from build123d import *

# Parameters (mm, degrees)
EXTRUDE_1_DEPTH     = 50
SKETCH_2_R          = 4
SKETCH_2_R_2        = 1.7
CUT_EXTRUDE_1_DEPTH = 50
SKETCH_3_W          = 10
SKETCH_3_H          = 10
EXTRUDE_2_DEPTH     = 2
FILLET_1_R          = 6
FILLET_2_R          = 6
FILLET_3_R          = 3
FILLET_4_R          = 3
SKETCH_5_R          = 1.5
CUT_EXTRUDE_2_DEPTH = 23
FILLET_5_R          = 2
FILLET_6_R          = 2
FILLET_7_R          = 2
FILLET_8_R          = 2
SKETCH_7_W          = 44.35766487
SKETCH_7_H          = 5
CUT_EXTRUDE_4_DEPTH = 5
CUT_EXTRUDE_5_DEPTH = 31


with BuildPart() as part:
    # 草图1 → 凸台-拉伸1 (new body)
    with BuildSketch(Plane.XY):
        Polygon((-45, 4.380640832), (-35, 4.380640832), (-35, -2.619359168), (-5, -2.619359168), (-5, 4.380640832), (5, 4.380640832), (5, -0.619359168), (0, -0.619359168), (0, -7.619359168), (-40, -7.619359168), (-40, -0.619359168), (-45, -0.619359168), align=None)
    extrude(amount=EXTRUDE_1_DEPTH)

    # 草图2 → 切除-拉伸1 (cut)
    with BuildSketch(Plane(origin=(0, -2.619359168, 0), x_dir=(1, 0, 0), z_dir=(0, 1, 0))):
        with Locations(Location((-20, -25, 0), (0, 0, 270))):
            Circle(SKETCH_2_R)
        with Locations(Location((-20, -17.75, 0), (0, 0, 270))):
            Circle(SKETCH_2_R_2)
        with Locations(Location((-12.75, -25, 0), (0, 0, 270))):
            Circle(SKETCH_2_R_2)
        with Locations(Location((-20, -32.25, 0), (0, 0, 270))):
            Circle(SKETCH_2_R_2)
        with Locations(Location((-27.25, -25, 0), (0, 0, 270))):
            Circle(SKETCH_2_R_2)
    extrude(amount=-CUT_EXTRUDE_1_DEPTH, mode=Mode.SUBTRACT)

    # 草图3 → 凸台-拉伸2 (add)
    with BuildSketch(Plane(origin=(0, 4.380640832, 0), x_dir=(1, 0, 0), z_dir=(0, 1, 0))):
        with Locations((0, -45)):
            Rectangle(SKETCH_3_W, SKETCH_3_H)
        with Locations((-40, -45)):
            Rectangle(SKETCH_3_W, SKETCH_3_H)
        with Locations((-40, -5)):
            Rectangle(SKETCH_3_W, SKETCH_3_H)
        with Locations((0, -5)):
            Rectangle(SKETCH_3_W, SKETCH_3_H)
    extrude(amount=EXTRUDE_2_DEPTH)

    # 圆角1
    fillet_1_edges = [part.edges().sort_by_distance(p)[0] for p in [
        (-40, -7.619359168, 25),
    ]]
    fillet(fillet_1_edges, radius=FILLET_1_R)

    # 圆角2
    fillet_2_edges = [part.edges().sort_by_distance(p)[0] for p in [
        (0, -7.619359168, 25),
    ]]
    fillet(fillet_2_edges, radius=FILLET_2_R)

    # 圆角3
    fillet_3_edges = [part.edges().sort_by_distance(p)[0] for p in [
        (-5, -2.619359168, 25),
    ]]
    fillet(fillet_3_edges, radius=FILLET_3_R)

    # 圆角4
    fillet_4_edges = [part.edges().sort_by_distance(p)[0] for p in [
        (-35, -2.619359168, 25),
    ]]
    fillet(fillet_4_edges, radius=FILLET_4_R)

    # 草图5 → 切除-拉伸2 (cut)
    with BuildSketch(Plane.XZ.offset(0.619359168)):
        with Locations((2.5, 47.5)):
            Circle(SKETCH_5_R)
        with Locations(Location((2.5, 2.5, 0), (0, 0, 270))):
            Circle(SKETCH_5_R)
        with Locations((-42.5, 2.5)):
            Circle(SKETCH_5_R)
        with Locations(Location((-42.5, 47.5, 0), (0, 0, 270))):
            Circle(SKETCH_5_R)
    extrude(amount=-CUT_EXTRUDE_2_DEPTH, mode=Mode.SUBTRACT)

    # 圆角5
    fillet_5_edges = [part.edges().sort_by_distance(p)[0] for p in [
        (5, 2.880640832, 50),
    ]]
    fillet(fillet_5_edges, radius=FILLET_5_R)

    # 圆角6
    fillet_6_edges = [part.edges().sort_by_distance(p)[0] for p in [
        (5, 2.880640832, 0),
    ]]
    fillet(fillet_6_edges, radius=FILLET_6_R)

    # 圆角7
    fillet_7_edges = [part.edges().sort_by_distance(p)[0] for p in [
        (-45, 2.880640832, 0),
    ]]
    fillet(fillet_7_edges, radius=FILLET_7_R)

    # 圆角8
    fillet_8_edges = [part.edges().sort_by_distance(p)[0] for p in [
        (-45, 2.880640832, 50),
    ]]
    fillet(fillet_8_edges, radius=FILLET_8_R)

    # 草图7 → 切除-拉伸4 (cut)
    with BuildSketch(Plane.XZ.offset(7.619359168)):
        with Locations((-20.290282059, 42.5)):
            Rectangle(SKETCH_7_W, SKETCH_7_H)
        with Locations((-20.290282059, 7.5)):
            Rectangle(SKETCH_7_W, SKETCH_7_H)
    extrude(amount=-CUT_EXTRUDE_4_DEPTH, mode=Mode.SUBTRACT)

    # 草图8 → 切除-拉伸5 (cut)
    with BuildSketch(Plane(origin=(0, 6.380640832, 0), x_dir=(1, 0, 0), z_dir=(0, 1, 0))):
        Polygon((-5, -40), (-8, -40), (-35, -40), (-35, -45), (-5, -45), align=None)
        Polygon((-35, -10), (-8, -10), (-5, -10), (-5, -5), (-35, -5), align=None)
    extrude(amount=-CUT_EXTRUDE_5_DEPTH, mode=Mode.SUBTRACT)


solid = part.part
Could you check a few things on this model? Use its own coordinates, in mm. A direction names the side the tool comes from. Give positions to 0.01 mm unless a question says otherwise; leave off trailing zeros. Order: outer loops, then holes, each group sorted by start corner. A loop starts at its lowest first (then second) coordinate and runs counter-clockwise, first axis right, second up. Notation, with made-up numbers: (20, 34.25) -> (61, 34.25) arc R24 ccw to (61, 44.25) -> close; hole circle Ø9 at (-12.5, 54.25). An arc over 180 degrees is marked (long way). Return JSON: item names as keys, results as strings.
1. Imagine slicing it at B-B on x = -12.75. List the corners of the cut face in (y, z) for me, then the cut area to 3 significant figures.
Answer list:
{"outline": "(-7.62, 0) -> (-2.62, 0) -> (-2.62, 5) -> (-7.62, 5) -> close; (-7.62, 10) -> (-2.62, 10) -> (-2.62, 23.3) -> (-7.62, 23.3) -> close; (-7.62, 26.7) -> (-2.62, 26.7) -> (-2.62, 40) -> (-7.62, 40) -> close; (-7.62, 45) -> (-2.62, 45) -> (-2.62, 50) -> (-7.62, 50) -> close", "area": "183 mm2"}
2. For pin 1 Ø5 at (x, z) = (-2, 30) entering from +Y; pin 2 Ø1 at (y, z) = (-4.5, 27.5) entering from +X; pin 3 Ø4 at (y, z) = (-6, 41.5) entering from +X, each with a flat end and sliding along its axis, tell me the tip position at first contact or that it passes through.
Answer list:
{"pin 1": "stops at y = 4.38", "pin 2": "stops at x = -0.49", "pin 3": "stops at x = -0.84"}
3. On a 3-axis mill with a long thin cutter (end or side, diameter ignored), from which of +Z, -Z, +X, -X, +Y, -Y can I reach the whole of each face in a straight line? I mean faces 4 (the flat face through (-42, -0.619, 25)), 5 (the flat face through (-40, 4.381, 25)), 6 (the cylindrical face through (-5.86, -1.72, 25.21)). Say none if no direction works.
Answer list:
{"face 4": "+Z, -Z, -X, -Y", "face 5": "+X, -X, +Y", "face 6": "+Z, -Z, +Y"}
4. Imagine slicing it at C-C on z = 25. List the corners of the cut face in (x, y) for me, then the cut area to 3 significant figures.
Answer list:
{"outline": "(-45, -0.62) -> (-40, -0.62) -> (-40, -1.62) arc R6 ccw to (-34, -7.62) -> (-28.95, -7.62) -> (-28.95, -2.62) -> (-32, -2.62) arc R3 cw to (-35, 0.38) -> (-35, 4.38) -> (-45, 4.38) -> close; (-25.55, -7.62) -> (-24, -7.62) -> (-24, -2.62) -> (-25.55, -2.62) -> close; (-16, -7.62) -> (-14.45, -7.62) -> (-14.45, -2.62) -> (-16, -2.62) -> close; (-11.05, -7.62) -> (-6, -7.62) arc R6 ccw to (0, -1.62) -> (0, -0.62) -> (5, -0.62) -> (5, 4.38) -> (-5, 4.38) -> (-5, 0.38) arc R3 cw to (-8, -2.62) -> (-11.05, -2.62) -> close", "area": "234 mm2"}
5. Imagine slicing it at A-A on y = 2.25. List the corners of the cut face in (x, z) for me.
Answer list:
{"outline": "(-45, 2) arc R2 ccw to (-43, 0) -> (-35, 0) -> (-35, 50) -> (-43, 50) arc R2 ccw to (-45, 48) -> close; (-5, 0) -> (3, 0) arc R2 ccw to (5, 2) -> (5, 48) arc R2 ccw to (3, 50) -> (-5, 50) -> close; hole circle Ø3 at (-42.5, 2.5); hole circle Ø3 at (-42.5, 47.5); hole circle Ø3 at (2.5, 2.5); hole circle Ø3 at (2.5, 47.5)"}
6. Imagine slicing it at D-D on x = -20. List the corners of the cut face in (y, z) for me.
Answer list:
{"outline": "(-7.62, 0) -> (-2.62, 0) -> (-2.62, 5) -> (-7.62, 5) -> close; (-7.62, 10) -> (-2.62, 10) -> (-2.62, 16.05) -> (-7.62, 16.05) -> close; (-7.62, 19.45) -> (-2.62, 19.45) -> (-2.62, 21) -> (-7.62, 21) -> close; (-7.62, 29) -> (-2.62, 29) -> (-2.62, 30.55) -> (-7.62, 30.55) -> close; (-7.62, 33.95) -> (-2.62, 33.95) -> (-2.62, 40) -> (-7.62, 40) -> close; (-7.62, 45) -> (-2.62, 45) -> (-2.62, 50) -> (-7.62, 50) -> close"}
7. Thinking about a two-plate mould opening in X: for faces 1 (the cylindrical face through (-44.4, 2.93, 0.57)), 2 (the flat face through (-40, 6.381, 45)), 3 (the cylindrical face through (-18.567, -5.084, 18.664)), which applies, pulls with the +X half, pulls with the -X half, needs draft (parallel to the pull), parting line crosses it, or undercut?
Answer list:
{"face 1": "pulls with the -X half", "face 2": "needs draft", "face 3": "undercut"}
8. I need wall thicknesses on line 1 (Z direction, x = -7.5, y = -4.25); line 2 (X direction, y = 0.75, z = 10.5); line 3 (X direction, y = 5.75, z = 48). Which ranges of each line are inside material? Lowest first, please. Write a range as from..to.
Answer list:
{"line 1": "z = 0..5, 10..40, 45..50", "line 2": "x = -45..-35, -5..5", "line 3": "x = -45..-43.91, -41.09..-35, -5..1.09, 3.91..5"}
